Autodesk Inventor part; units mm, degrees
ref_plane "YZ Plane" through (0, 0, 0) normal (1, 0, 0) x (0, 1, 0)
ref_plane "XZ Plane" through (0, 0, 0) normal (0, 1, 0) x (-1, 0, 0)
ref_plane "XY Plane" through (0, 0, 0) normal (0, 0, 1) x (1, 0, 0)
sketch "Эскиз1" plane through (0, 0, 0) normal (0, 0, 1) x (1, 0, 0)
  circle A0 centre (0, 0) radius 2
  dimension "d0" = 4
extrude "Выдавливание1" add sketch "Эскиз1" along normal blind 98
sketch "Эскиз2" plane through (0, 0, 98) normal (0, 0, 1) x (1, 0, 0)
  line L0 (0, 3.7538) -> (3.2509, 1.8769)
  line L1 (3.2509, 1.8769) -> (3.2509, -1.8769)
  line L2 (3.2509, -1.8769) -> (0, -3.7538)
  line L3 (0, -3.7538) -> (-3.2509, -1.8769)
  line L4 (-3.2509, -1.8769) -> (-3.2509, 1.8769)
  line L5 (-3.2509, 1.8769) -> (0, 3.7538)
  point P0 (0, 0)
  point P1 (0, 0)
extrude "Выдавливание2" add sketch "Эскиз2" along normal blind 5.5
sketch "Эскиз3" plane through (0, 0, 103.5) normal (0, 0, 1) x (1, 0, 0)
  circle A0 centre (0, 0) radius 2
  circle A1 centre (0, 0) radius 2
extrude "Выдавливание3" add sketch "Эскиз3" along normal blind 5
thread "Резьба1"
mirror "Зеркальное отражение1" about plane through (0, 0, 0) normal (0, 0, -1)
properties part number "ось пушки 3" material "Сталь, литейная"
Read the model definition and answer for the solid it produces. Units are mm, in the model's axes. A direction names the side the tool comes from. Give positions to 0.01 mm unless a question says otherwise; leave off trailing zeros. Write each loop counter-clockwise with the first axis right and the second up, starting at its lowest first coordinate (ties: lowest second). Pieces come first, ordered by that corner, then holes. Notation, with made-up numbers: (-23.5, 71) - (18.5, 71) arc R32 cw to (18.5, 103) - close; hole circle Ø10 at (56.5, -12.75). An arc over 180 degrees is marked (long way). Use CSV: the item, a comma, the result in double quotes. Start each with the question number.
(1) For faces 1 (the flat face through (-1, -2, 103.5)), 2 (the cylindrical face through (0, 2, -1)), 3 (the flat face through (1, -2, -103.5)), determine the directions among +Z, -Z, +X, -X, +Y, -Y from which every point of the face is accessible in a straight line to the end or side of a thin tool.
(2) Consider line 1 along Z through (x, y) = (0, -3); line 2 along Y through (x, z) = (0.25, 2); line 3 along Y through (x, z) = (-0.75, -60). Determine where each line is inside the solid, lowest interval first.
(3) Given P1, Ø1, axis at x = 1.5, y = -2.5, coming from the +Z side; P2, Ø3, axis at x = 0.5, z = -47.5, coming from the +Y side; P3, Ø1, axis at y = 2, z = -33.5, coming from the -X side; P4, Ø1, axis at y = -3, z = 48, coming from the -X side, each flat-ended and moving along its own axis, determine where each tip first touches the part or whether it passes through.
(4) Find section B-B (z = -57). Give the vertices of the cut face in (x, y), plus the area to 3 significant figures.
(5) Find section A-A (y = 0). Give the vertices of the cut face in (x, z).
Findings below:
1,face 1,"+Z"
1,face 2,"none"
1,face 3,"-Z"
2,line 1,"-103.5 to -98, 98 to 103.5"
2,line 2,"-1.98 to 1.98"
2,line 3,"-1.85 to 1.85"
3,P1,"z = 103.5"
3,P2,"y = 2"
3,P3,"x = -1.32"
3,P4,"through"
4,outline,"circle Ø4 at (0, 0)"
4,area,"12.6 mm2"
5,outline,"(-3.25, -103.5) - (-2, -103.5) - (-2, -108.5) - (2, -108.5) - (2, -103.5) - (3.25, -103.5) - (3.25, -98) - (2, -98) - (2, 98) - (3.25, 98) - (3.25, 103.5) - (2, 103.5) - (2, 108.5) - (-2, 108.5) - (-2, 103.5) - (-3.25, 103.5) - (-3.25, 98) - (-2, 98) - (-2, -98) - (-3.25, -98) - close"
